Input: part model. Units: mm. Frame: model coordinates. A direction names the side the tool comes from. Coordinates: 2 decimals unless noted, no trailing zeros. Loops run counter-clockwise (first coordinate to the right, second up) from the corner with the lowest first, then second, coordinate; pieces in that order, holes last. Notation, with made-up numbers: M 6,89.25 L 58,89.25 A19 ccw 58,111.25 Z; hole C 60.25,10.25 d5. An arc over 180 degrees is marked long. Use a Markdown table: item, result. Add a question column.
1. Pin query (flat end, axial travel): pin 1 (4 mm diameter, centred on x = -87, z = 115, fed in from -Y); pin 2 (10 mm diameter, centred on y = 50, z = 106.5, fed in from -X); pin 3 (12 mm diameter, centred on y = -56, z = 124.5, fed in from +X). Return the tip coordinate at first contact, or that it passes through.
2. Section A-A on x = 0. Output: boundary loops of the cut face in (y, z).
3. Draft query along Y for faces 4 (the cylindrical face through (33, -56, 87)), 5 (the cylindrical face through (159.804, -108.789, 86.275)), 6 (the flat face through (118, 63, 175)). Return one class per face: +Y half, -Y half, draft (parallel to the pull), parting line (faces both ways), or undercut.
4. Set-up query: faces 1 (the flat face through (106, -81, 175)), 2 (the flat face through (-108, 83, 175)), 3 (the flat face through (106, -81, 0)). Return all of +Z, -Z, +X, -X, +Y, -Y with unobstructed straight access to the full face (end or side cutting, diameter ignored); none if empty.
5. Section B-B on y = -104.5. State how many separate pieces and enclosed holes the cut face has, then the cut area to 3 significant figures.
6. Line query: L1, parallel to X at y = 94, z = 60.5; L2, parallel to X at y = 90, z = 46.5; L3, parallel to Y at x = 45, z = 141.5. Output: solid intervals per line, ascending. Write a range as [from, to].
Autodesk Inventor part; units mm, degrees
ref_plane "Work Plane1" through (0, 0, 87.5) normal (0, 0, 1) x (1, 0, 0)
ref_plane "YZ Plane" through (0, 0, 0) normal (1, 0, 0) x (0, 1, 0)
ref_plane "XZ Plane" through (0, 0, 0) normal (0, 1, 0) x (-1, 0, 0)
sketch "Sketch2" plane through (0, 0, 0) normal (0, 0, 1) x (1, 0, 0)
  point P0 (0, 0)
ref_plane "Work Plane1" through (0, 0, 87.5) normal (0, 0, 1) x (1, 0, 0)
sketch "Sketch3" plane through (0, 0, 87.5) normal (0, 0, 1) x (1, 0, 0)
  circle A0 centre (0, 0) radius 65
  circle A1 centre (0, 50) radius 5
  circle A2 centre (-47.5528, 15.4508) radius 5
  circle A3 centre (-29.3893, -40.4508) radius 5
  circle A4 centre (29.3893, -40.4508) radius 5
  circle A5 centre (47.5528, 15.4508) radius 5
  dimension "d11" = 130
  dimension "d33" = 10
  dimension "d36" = 360
sketch "Sketch5" plane through (0, 0, 0) normal (0, 0, 1) x (1, 0, 0)
  circle A0 centre (0, 0) radius 30
  circle A1 centre (0, 0) radius 190.5
  line L0 (6.509, 17.129) -> (57.211, 63.0349) construction
  line L1 (57.211, 63.0349) -> (22.2678, 145.9394) construction
  line L2 (22.2678, 145.9394) -> (41.4523, 171.2904) construction
  line L3 (41.4523, 171.2904) -> (59.2665, 184.9937) construction
  spline S0 degree 4 poles (6.509, 17.129) (57.211, 63.0349) (22.2678, 145.9394) (41.4523, 171.2904) (59.2665, 184.9937) knots 1 1 1 1 1 2 2 2 2 2
  line L4 (0, 17.129) -> (-30, 60.9794) construction
  line L5 (-30, 60.9794) -> (0, 136.3472) construction
  line L6 (0, 136.3472) -> (-6.509, 176.0866) construction
  line L7 (-6.509, 176.0866) -> (-30, 190.5) construction
  spline S1 degree 4 poles (0, 17.129) (-30, 60.9794) (0, 136.3472) (-6.509, 176.0866) (-30, 190.5) knots 1 1 1 1 1 2 2 2 2 2
  line L8 (0, 17.129) -> (6.509, 17.129)
  arc A2 (59.2665, 184.9937) -> (-30, 190.5) centre (2.5103, -8.7844) ccw
  line L9 (-11.5797, 14.2015) -> (-25.9843, 81.0636) construction
  line L10 (-25.9843, 81.0636) -> (-115.2534, 92.2542) construction
  line L11 (-115.2534, 92.2542) -> (-127.6157, 121.5439) construction
  line L12 (-127.6157, 121.5439) -> (-130.576, 143.8231) construction
  spline S2 degree 4 poles (-11.5797, 14.2015) (-25.9843, 81.0636) (-115.2534, 92.2542) (-127.6157, 121.5439) (-130.576, 143.8231) knots 1 1 1 1 1 2 2 2 2 2
  line L13 (-14.8342, 8.5645) -> (-67.8097, 4.5089) construction
  line L14 (-67.8097, 4.5089) -> (-118.0801, 68.1736) construction
  line L15 (-118.0801, 68.1736) -> (-155.7499, 82.4063) construction
  line L16 (-155.7499, 82.4063) -> (-179.9778, 69.2692) construction
  spline S3 degree 4 poles (-14.8342, 8.5645) (-67.8097, 4.5089) (-118.0801, 68.1736) (-155.7499, 82.4063) (-179.9778, 69.2692) knots 1 1 1 1 1 2 2 2 2 2
  line L17 (-14.8342, 8.5645) -> (-11.5797, 14.2015)
  arc A3 (-130.576, 143.8231) -> (-179.9778, 69.2692) centre (8.8627, -2.2182) ccw
  line L18 (-18.0887, -2.9275) -> (-83.1953, 18.0287) construction
  line L19 (-83.1953, 18.0287) -> (-137.5211, -53.6853) construction
  line L20 (-137.5211, -53.6853) -> (-169.068, -49.7465) construction
  line L21 (-169.068, -49.7465) -> (-189.8425, -41.1705) construction
  spline S4 degree 4 poles (-18.0887, -2.9275) (-83.1953, 18.0287) (-137.5211, -53.6853) (-169.068, -49.7465) (-189.8425, -41.1705) knots 1 1 1 1 1 2 2 2 2 2
  line L22 (-14.8342, -8.5645) -> (-37.8097, -56.4705) construction
  line L23 (-37.8097, -56.4705) -> (-118.0801, -68.1736) construction
  line L24 (-118.0801, -68.1736) -> (-149.2409, -93.6803) construction
  line L25 (-149.2409, -93.6803) -> (-149.9778, -121.2308) construction
  spline S5 degree 4 poles (-14.8342, -8.5645) (-37.8097, -56.4705) (-118.0801, -68.1736) (-149.2409, -93.6803) (-149.9778, -121.2308) knots 1 1 1 1 1 2 2 2 2 2
  line L26 (-14.8342, -8.5645) -> (-18.0887, -2.9275)
  arc A4 (-189.8425, -41.1705) -> (-149.9778, -121.2308) centre (6.3524, 6.5662) ccw
  line L27 (-6.509, -17.129) -> (-57.211, -63.0349) construction
  line L28 (-57.211, -63.0349) -> (-22.2678, -145.9394) construction
  line L29 (-22.2678, -145.9394) -> (-41.4523, -171.2904) construction
  line L30 (-41.4523, -171.2904) -> (-59.2665, -184.9937) construction
  spline S6 degree 4 poles (-6.509, -17.129) (-57.211, -63.0349) (-22.2678, -145.9394) (-41.4523, -171.2904) (-59.2665, -184.9937) knots 1 1 1 1 1 2 2 2 2 2
  line L31 (0, -17.129) -> (30, -60.9794) construction
  line L32 (30, -60.9794) -> (0, -136.3472) construction
  line L33 (0, -136.3472) -> (6.509, -176.0866) construction
  line L34 (6.509, -176.0866) -> (30, -190.5) construction
  spline S7 degree 4 poles (0, -17.129) (30, -60.9794) (0, -136.3472) (6.509, -176.0866) (30, -190.5) knots 1 1 1 1 1 2 2 2 2 2
  line L35 (0, -17.129) -> (-6.509, -17.129)
  arc A5 (-59.2665, -184.9937) -> (30, -190.5) centre (-2.5103, 8.7844) ccw
  line L36 (11.5797, -14.2015) -> (25.9843, -81.0636) construction
  line L37 (25.9843, -81.0636) -> (115.2534, -92.2542) construction
  line L38 (115.2534, -92.2542) -> (127.6157, -121.5439) construction
  line L39 (127.6157, -121.5439) -> (130.576, -143.8231) construction
  spline S8 degree 4 poles (11.5797, -14.2015) (25.9843, -81.0636) (115.2534, -92.2542) (127.6157, -121.5439) (130.576, -143.8231) knots 1 1 1 1 1 2 2 2 2 2
  line L40 (14.8342, -8.5645) -> (67.8097, -4.5089) construction
  line L41 (67.8097, -4.5089) -> (118.0801, -68.1736) construction
  line L42 (118.0801, -68.1736) -> (155.7499, -82.4063) construction
  line L43 (155.7499, -82.4063) -> (179.9778, -69.2692) construction
  spline S9 degree 4 poles (14.8342, -8.5645) (67.8097, -4.5089) (118.0801, -68.1736) (155.7499, -82.4063) (179.9778, -69.2692) knots 1 1 1 1 1 2 2 2 2 2
  line L44 (14.8342, -8.5645) -> (11.5797, -14.2015)
  arc A6 (130.576, -143.8231) -> (179.9778, -69.2692) centre (-8.8627, 2.2182) ccw
  line L45 (18.0887, 2.9275) -> (83.1953, -18.0287) construction
  line L46 (83.1953, -18.0287) -> (137.5211, 53.6853) construction
  line L47 (137.5211, 53.6853) -> (169.068, 49.7465) construction
  line L48 (169.068, 49.7465) -> (189.8425, 41.1705) construction
  spline S10 degree 4 poles (18.0887, 2.9275) (83.1953, -18.0287) (137.5211, 53.6853) (169.068, 49.7465) (189.8425, 41.1705) knots 1 1 1 1 1 2 2 2 2 2
  line L49 (14.8342, 8.5645) -> (37.8097, 56.4705) construction
  line L50 (37.8097, 56.4705) -> (118.0801, 68.1736) construction
  line L51 (118.0801, 68.1736) -> (149.2409, 93.6803) construction
  line L52 (149.2409, 93.6803) -> (149.9778, 121.2308) construction
  spline S11 degree 4 poles (14.8342, 8.5645) (37.8097, 56.4705) (118.0801, 68.1736) (149.2409, 93.6803) (149.9778, 121.2308) knots 1 1 1 1 1 2 2 2 2 2
  line L53 (14.8342, 8.5645) -> (18.0887, 2.9275)
  arc A7 (189.8425, 41.1705) -> (149.9778, 121.2308) centre (-6.3524, -6.5662) ccw
  dimension "d24" = 60
  dimension "d25" = 381
  dimension "d28" = 360
extrude "Extrusion4" add sketch "Sketch5" along normal blind 175 contours S10 L53 S11 A0 | A0 S11 A1 S10 | S9 A1 S8 A0 | A0 S8 L44 S9 | A1 S11 A7 S10 | S9 A6 S8 A1 | S0 L8 S1 A0 | A0 S1 A1 S0 | S7 A1 S6 A0 | A0 S6 L35 S7 | A1 S1 A2 S0 | S7 A5 S6 A1 | S2 L17 S3 A0 | A0 S3 A1 S2 | S5 A1 S4 A0 | A0 S4 L26 S5 | A1 S3 A3 S2 | S5 A4 S4 A1
extrude "Extrusion5" add sketch "Sketch3" along normal mid plane 180
sketch "Sketch6" plane through (0, 0, -2.5) normal (0, 0, -1) x (-1, 0, 0)
  circle A0 centre (-47.5528, 15.4508) radius 5
  circle A1 centre (-29.3893, -40.4508) radius 5
  circle A2 centre (29.3893, -40.4508) radius 5
  circle A3 centre (47.5528, 15.4508) radius 5
  circle A4 centre (0, 50) radius 5
  circle A5 centre (0, 0) radius 65
  circle A6 centre (0, 50) radius 5
  circle A7 centre (-47.5528, 15.4508) radius 5
  circle A8 centre (-29.3893, -40.4508) radius 5
  circle A9 centre (29.3893, -40.4508) radius 5
  circle A10 centre (47.5528, 15.4508) radius 5
  dimension "d42" = 360
extrude "Extrusion6" cut sketch "Sketch6" against normal blind 1800 contours A0 | A1 | A2 | A3 | A4
properties part number "velg" material "Aluminum 6061"
Answers below:
| question | item | result |
|---|---|---|
| 1 | pin 1 | stops at y = -64.92 |
| 1 | pin 2 | stops at x = -116.88 |
| 1 | pin 3 | stops at x = 128.89 |
| 2 | outline | M -193.12,0 L -65,0 L -65,-2.5 L 45,-2.5 L 45,177.5 L -65,177.5 L -65,175 L -193.12,175 Z; M 55,-2.5 L 65,-2.5 L 65,0 L 193.12,0 L 193.12,175 L 65,175 L 65,177.5 L 55,177.5 Z |
| 3 | face 4 | undercut |
| 3 | face 5 | -Y half |
| 3 | face 6 | draft |
| 4 | face 1 | +Z, +X, -Y |
| 4 | face 2 | +Z, -X, +Y |
| 4 | face 3 | -Z, +X, -Y |
| 5 | separate pieces | 3 |
| 5 | enclosed holes | 0 |
| 5 | area | 21,700 mm² |
| 6 | L1 | x = [-168.66, -88.78], [-12.58, 35.55], [136.18, 168.74] |
| 6 | L2 | x = [-170.77, -82.54], [-12.77, 35.25], [131.61, 170.98] |
| 6 | L3 | y = [-64.06, 11.15], [19.75, 46.9], [167.72, 188.61] |
